Check sheet for the modelled part. Datum: model origin and axes. Units: mm. Round coordinates to 2 decimals unless told otherwise and drop trailing zeros. Order: outer loops, then holes, each group sorted by start corner. A loop starts at its lowest first (then second) coordinate and runs counter-clockwise, first axis right, second up. Notation, with made-up numbers: (61, 1) -> (113, 1) arc R18 ccw to (113, 19) -> close; hole circle Ø3 at (65, 70). An arc over 180 degrees is marked (long way). Answer in a Markdown table with one row per item.
Autodesk Inventor part; units mm, degrees
ref_plane "YZ Plane" through (0, 0, 0) normal (1, 0, 0) x (0, 1, 0)
ref_plane "XZ Plane" through (0, 0, 0) normal (0, 1, 0) x (-1, 0, 0)
ref_plane "XY Plane" through (0, 0, 0) normal (0, 0, 1) x (1, 0, 0)
sketch "Esboço1" plane through (0, 0, 0) normal (0, 0, 1) x (1, 0, 0)
  circle A0 centre (0, 0) radius 8
  dimension "d0" = 16
extrude "Extrusão1" add sketch "Esboço1" along normal blind 1014.5
sketch "Esboço2" plane through (0, 0, 1014.5) normal (0, 0, 1) x (1, 0, 0)
  circle A0 centre (0, 0) radius 6
  dimension "d3" = 12
extrude "Extrusão2" add sketch "Esboço2" along normal blind 39
sketch "Esboço3" plane through (0, 0, 1053.5) normal (0, 0, 1) x (1, 0, 0)
  circle A0 centre (0, 0) radius 5
  dimension "d6" = 10
extrude "Extrusão3" add sketch "Esboço3" along normal blind 15
sketch "Esboço4" plane through (0, 0, 0) normal (0, 0, -1) x (-1, 0, 0)
  circle A0 centre (0, 0) radius 5
  dimension "d9" = 10
extrude "Extrusão4" add sketch "Esboço4" along normal blind 9.15
sketch "Esboço5" plane through (0, 0, -9.15) normal (0, 0, -1) x (-1, 0, 0)
  circle A0 centre (0, 0) radius 4.5
  dimension "d12" = 9
extrude "Extrusão5" add sketch "Esboço5" along normal blind 1.15
sketch "Esboço6" plane through (0, 0, -10.3) normal (0, 0, -1) x (-1, 0, 0)
  circle A0 centre (0, 0) radius 5
  dimension "d15" = 10
extrude "Extrusão6" add sketch "Esboço6" along normal blind 1.85
thread "Rosca1"
chamfer "Chanfro1" distance 0.5 angle 45 5 edges at (-5, 0, 1068.5) (-6, 0, 1053.5) (-8, 0, 1014.5) (-8, 0, 0) (5, 0, -12.15)
properties part number "SFU16XX_Y2"
(1) Section check C-C on z = 68.5. Record the boundary of the cut face in (x, y).
Solutions:
| item | result |
|---|---|
| outline | circle Ø16 at (0, 0) |
(2) Depth check by flat-ended pin: pin 1 Ø8 at (y, z) = (-2, 445) entering from -X; pin 2 Ø3 at (y, z) = (2, 432) entering from +X; pin 3 Ø2 at (x, z) = (-3, 649) entering from -Y; pin 4 Ø1.5 at (x, z) = (2, 287.5) entering from +Y. Enter the tip coordinate at first touch or a pass-through.
Solutions:
| item | result |
|---|---|
| pin 1 | x = -8 |
| pin 2 | x = 7.98 |
| pin 3 | y = -7.75 |
| pin 4 | y = 7.9 |
(3) Scan lines: probe 1 along Z at (x, y) = (7, -0.75); probe 2 along Z at (x, y) = (-6.75, -4); probe 3 along Y at (x, z) = (-1.25, 480.5). Record each from-to range of solid material in increasing order. Write a range as from..to.
Solutions:
| item | result |
|---|---|
| probe 1 | 0..1014.5 |
| probe 2 | 0.35..1014.15 |
| probe 3 | -7.9..7.9 |
